Build history of the part. All positions in model axes, mm. Face numbers are marked on the shaded views. Give positions to 0.01 mm unless a question says otherwise; leave off trailing zeros. Order: outer loops, then holes, each group sorted by start corner. A loop starts at its lowest first (then second) coordinate and runs counter-clockwise, first axis right, second up. Notation, with made-up numbers: (5, 58.5) -> (51, 58.5) arc R23 cw to (51, 97.5) -> close; hole circle Ø7 at (81, 52). An arc over 180 degrees is marked (long way). One line per question, with ' | ' between items. Start each with the question number.
(1) Pull direction Z, two halves, no side cores. Call the marked faces 1 and 2: +Z half, -Z half, draft (parallel to the pull), parting line (faces both ways), or undercut.
(2) Cut at A-A (y = 8.5). Give the cut face in (x, z), then the cut area to 3 significant figures.
(3) Cut at C-C (y = 17). Give the cut face in (x, z).
(4) Cut at D-D (z = -20). Give the cut face in (x, y), then the cut area to 3 significant figures.
(5) Drill centre lines: L1, parallel to X at y = 6.5, z = -35.5; L2, parallel to Z at x = -18, y = 4; L3, parallel to X at y = 18.5, z = -81. Where is each one in solid material? Low to high. Write a range as from..to.
(6) Cut at B-B (x = -71). Give the cut face in (y, z).
(7) Pin check, flat tips, straight feed: pin 1 Ø3 at (x, y) = (-17.5, 5.5) entering from +Z; pin 2 Ø10 at (y, z) = (22, -104) entering from +X; pin 3 Ø1.9 at (x, z) = (-84, -85) entering from +Y. Stop position of each tip, or through.
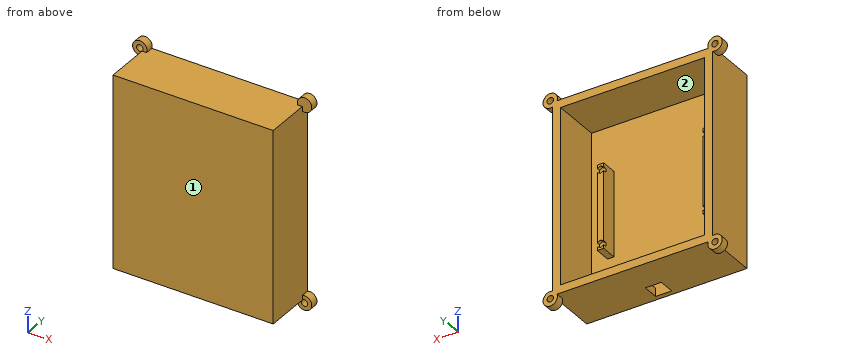
Autodesk Inventor part; units mm, degrees
ref_plane "YZ Plane" through (0, 0, 0) normal (1, 0, 0) x (0, 1, 0)
ref_plane "XZ Plane" through (0, 0, 0) normal (0, 1, 0) x (-1, 0, 0)
ref_plane "XY Plane" through (0, 0, 0) normal (0, 0, 1) x (1, 0, 0)
sketch "Sketch2" plane through (0, 0, 0) normal (0, 1, 0) x (-1, 0, 0)
  line L0 (0, 0) -> (100, 0)
  line L1 (100, 0) -> (100, -120)
  line L2 (100, -120) -> (0, -120)
  line L3 (0, -120) -> (0, 0)
  dimension "d0" = 100
  dimension "d1" = 120
extrude "Extrusion1" add sketch "Sketch2" along normal blind 3
sketch "Sketch3" plane through (0, 3, 0) normal (0, 1, 0) x (1, 0, 0)
  line L0 (0, 120) -> (-100, 120)
  line L1 (-100, 120) -> (-100, 0)
  line L2 (-95, 115) -> (-5, 115)
  line L3 (-5, 115) -> (-5, 5)
  line L4 (-5, 5) -> (-95, 5)
  line L5 (-95, 5) -> (-95, 115)
  line L6 (-100, 120) -> (0, 120)
  line L7 (0, 120) -> (0, 0)
  line L8 (0, 0) -> (-100, 0)
  line L9 (-100, 0) -> (-100, 120)
  dimension "d6" = 90
  dimension "d7" = 110
extrude "Extrusion2" add sketch "Sketch3" along normal blind 30
sketch "Sketch4" plane through (0, 3, 0) normal (0, 1, 0) x (1, 0, 0)
  line L0 (-95, 115) -> (-95, 5)
  line L1 (-95, 115) -> (-95, 85)
  line L2 (-85, 85) -> (-15, 85)
  line L3 (-15, 85) -> (-15, 35)
  line L4 (-15, 35) -> (-85, 35)
  line L5 (-85, 35) -> (-85, 85)
  line L6 (-85, 85) -> (-81, 85)
  line L7 (-81, 85) -> (-81, 35)
  line L8 (-81, 35) -> (-85, 35)
  line L9 (-85, 35) -> (-85, 85)
  line L10 (-15, 85) -> (-19, 85)
  line L11 (-19, 85) -> (-19, 35)
  line L12 (-19, 35) -> (-15, 35)
  line L13 (-15, 35) -> (-15, 85)
  line L14 (-85, 85) -> (-81, 85)
  line L15 (-81, 85) -> (-81, 81)
  line L16 (-81, 81) -> (-85, 81)
  line L17 (-85, 81) -> (-85, 85)
  line L18 (-85, 35) -> (-81, 35)
  line L19 (-81, 35) -> (-81, 39)
  line L20 (-81, 39) -> (-85, 39)
  line L21 (-85, 39) -> (-85, 35)
  line L22 (-19, 35) -> (-15, 35)
  line L23 (-15, 35) -> (-15, 39)
  line L24 (-15, 39) -> (-19, 39)
  line L25 (-19, 39) -> (-19, 35)
  line L26 (-19, 85) -> (-15, 85)
  line L27 (-15, 85) -> (-15, 81)
  line L28 (-15, 81) -> (-19, 81)
  line L29 (-19, 81) -> (-19, 85)
  circle A0 centre (-83, 83) radius 1
  circle A1 centre (-83, 37) radius 1
  circle A2 centre (-17, 37) radius 1
  circle A3 centre (-17, 83) radius 1
  point P0 (0, 0)
  dimension "d12" = 70
  dimension "d13" = 50
  dimension "d14" = 4
  dimension "d15" = 4
  dimension "d16" = 4
  dimension "d17" = 4
  dimension "d18" = 2
  dimension "d19" = 2
  dimension "d20" = 2
sketch "Sketch5" plane through (0, 33, 0) normal (0, 1, 0) x (1, 0, 0)
  point P0 (0, 0)
sketch "Sketch6" plane through (0, 33, 0) normal (0, 1, 0) x (1, 0, 0)
  line L0 (-100, 0) -> (0, 0)
  line L1 (0, 0) -> (10, 0) construction
  circle A0 centre (1.4142, -1.4142) radius 2
  circle A1 centre (1.4142, -1.4142) radius 4.5
  circle A2 centre (1.4084, 121.4127) radius 2
  circle A3 centre (1.4084, 121.4127) radius 4.5
  circle A4 centre (-101.4585, 121.4298) radius 2
  circle A5 centre (-101.4585, 121.4298) radius 4.5
  circle A6 centre (-101.4195, -1.4184) radius 2
  circle A7 centre (-101.4195, -1.4184) radius 4.5
  dimension "d24" = 4
  dimension "d25" = 9
  dimension "d27" = 4
  dimension "d28" = 9
  dimension "d30" = 4
  dimension "d31" = 9
  dimension "d33" = 4
  dimension "d34" = 9
extrude "Extrusion3" add sketch "Sketch6" against normal blind 5
extrude "Extrusion4" add sketch "Sketch4" along normal blind 10 contours L16 L7 L20 L5 | L28 L3 L24 L11
sketch "Sketch7" plane through (0, 13, 0) normal (0, 1, 0) x (1, 0, 0)
  point P0 (0, 0)
sketch "Sketch10" plane through (0, 13, 0) normal (0, 1, 0) x (1, 0, 0)
  line L0 (-81, 81) -> (-85, 81)
  line L1 (-81, 39) -> (-81, 81)
  line L2 (-85, 81) -> (-81, 81)
  line L3 (-81, 81) -> (-81, 39)
  line L4 (-81, 39) -> (-85, 39)
  line L5 (-85, 39) -> (-85, 81)
  point P0 (0, 0)
sketch "Sketch11" plane through (0, 13, 0) normal (0, 1, 0) x (1, 0, 0)
  line L0 (-15, 81) -> (-19, 81)
  line L1 (-15, 39) -> (-15, 81)
  line L2 (-19, 81) -> (-15, 81)
  line L3 (-15, 81) -> (-15, 39)
  line L4 (-15, 39) -> (-19, 39)
  line L5 (-19, 39) -> (-19, 81)
  line L6 (-85, 81) -> (-81, 81)
  line L7 (-85, 81) -> (-81, 81)
  line L8 (-81, 81) -> (-81, 85)
  line L9 (-81, 85) -> (-85, 85)
  line L10 (-85, 85) -> (-85, 81)
  line L11 (-19, 39) -> (-19, 81)
  line L12 (-19, 81) -> (-15, 81)
  line L13 (-15, 81) -> (-15, 85)
  line L14 (-15, 85) -> (-19, 85)
  line L15 (-19, 85) -> (-19, 81)
  line L16 (-15, 39) -> (-19, 39)
  line L17 (-19, 39) -> (-15, 39)
  line L18 (-15, 39) -> (-15, 35)
  line L19 (-15, 35) -> (-19, 35)
  line L20 (-19, 35) -> (-19, 39)
  line L21 (-85, 39) -> (-81, 39)
  line L22 (-81, 39) -> (-81, 35)
  line L23 (-81, 35) -> (-85, 35)
  line L24 (-85, 35) -> (-85, 39)
  circle A0 centre (-83, 83) radius 1
  circle A1 centre (-17, 83) radius 1
  circle A2 centre (-17, 37) radius 1
  circle A3 centre (-83, 37) radius 1
  line L25 (-19, 84.1547) -> (-17, 85.3094)
  line L26 (-17, 85.3094) -> (-15, 84.1547)
  line L27 (-15, 84.1547) -> (-15, 81.8453)
  line L28 (-15, 81.8453) -> (-17, 80.6906)
  line L29 (-17, 80.6906) -> (-19, 81.8453)
  line L30 (-19, 81.8453) -> (-19, 84.1547)
  line L31 (-19, 38.1547) -> (-17, 39.3094)
  line L32 (-17, 39.3094) -> (-15, 38.1547)
  line L33 (-15, 38.1547) -> (-15, 35.8453)
  line L34 (-15, 35.8453) -> (-17, 34.6906)
  line L35 (-17, 34.6906) -> (-19, 35.8453)
  line L36 (-19, 35.8453) -> (-19, 38.1547)
  line L37 (-81, 35.8453) -> (-83, 34.6906)
  line L38 (-83, 34.6906) -> (-85, 35.8453)
  line L39 (-85, 35.8453) -> (-85, 38.1547)
  line L40 (-85, 38.1547) -> (-83, 39.3094)
  line L41 (-83, 39.3094) -> (-81, 38.1547)
  line L42 (-81, 38.1547) -> (-81, 35.8453)
  line L43 (-81, 81.8453) -> (-83, 80.6906)
  line L44 (-83, 80.6906) -> (-85, 81.8453)
  line L45 (-85, 81.8453) -> (-85, 84.1547)
  line L46 (-85, 84.1547) -> (-83, 85.3094)
  line L47 (-83, 85.3094) -> (-81, 84.1547)
  line L48 (-81, 84.1547) -> (-81, 81.8453)
  point P0 (0, 0)
  point P1 (-19, 83)
  point P2 (-19, 37)
  point P3 (-81, 37)
  point P4 (-81, 83)
  dimension "d75" = 4
  dimension "d76" = 4
  dimension "d77" = 2
  dimension "d78" = 2
  dimension "d79" = 2
sketch "Sketch17" plane through (0, 3, 0) normal (0, 1, 0) x (1, 0, 0)
  line L0 (-85, 85) -> (-15, 85)
  line L1 (-15, 85) -> (-15, 35)
  line L2 (-15, 35) -> (-85, 35)
  line L3 (-85, 35) -> (-85, 85)
  line L4 (-85, 85) -> (-81, 85)
  line L5 (-81, 85) -> (-81, 35)
  line L6 (-81, 35) -> (-85, 35)
  line L7 (-85, 35) -> (-85, 85)
  line L8 (-15, 85) -> (-19, 85)
  line L9 (-19, 85) -> (-19, 35)
  line L10 (-19, 35) -> (-15, 35)
  line L11 (-15, 35) -> (-15, 85)
  point P0 (0, 0)
  point P1 (-95, 115)
extrude "Extrusion7" add sketch "Sketch17" along normal blind 10 contours L0 L5 L2 L3 | L0 L1 L2 L9
sketch "Sketch18" plane through (0, 3, 0) normal (0, 1, 0) x (1, 0, 0)
  line L0 (-19, 35) -> (-19, 85)
  line L1 (-19, 35) -> (-15, 35)
  line L2 (-15, 35) -> (-15, 33.5)
  line L3 (-15, 33.5) -> (-19, 33.5)
  line L4 (-19, 33.5) -> (-19, 35)
  line L5 (-19, 85) -> (-15, 85)
  line L6 (-15, 85) -> (-15, 86.5)
  line L7 (-15, 86.5) -> (-19, 86.5)
  line L8 (-19, 86.5) -> (-19, 85)
  line L9 (-81, 85) -> (-85, 85)
  line L10 (-85, 85) -> (-81, 85)
  line L11 (-81, 85) -> (-81, 86.5)
  line L12 (-81, 86.5) -> (-85, 86.5)
  line L13 (-85, 86.5) -> (-85, 85)
  line L14 (-85, 35) -> (-81, 35)
  line L15 (-85, 35) -> (-81, 35)
  line L16 (-81, 35) -> (-81, 33.5)
  line L17 (-81, 33.5) -> (-85, 33.5)
  line L18 (-85, 33.5) -> (-85, 35)
  point P0 (0, 0)
  dimension "d80" = 4
  dimension "d81" = 1.5
  dimension "d82" = 1.5
extrude "Extrusion8" add sketch "Sketch18" along normal blind 10
extrude "Extrusion9" cut sketch "Sketch11" against normal blind 2 contours L28 L29 L0 | L0 L29 L15 L25 L14 L26 L13 L28 | L32 L18 L34 L19 L35 L20 L31 L4 | L4 L31 L32 | L14 L25 L26 | L34 L35 L19 | L44 L10 L46 L9 L47 L8 L43 L6 | L6 L43 L44 | L46 L47 L9 | L40 L41 L21 | L21 L41 L22 L37 L23 L38 L24 L40 | L23 L37 L38 | A0 | A1 | A2 | A3
sketch "Sketch19" plane through (0, 28, 0) normal (0, -1, 0) x (1, 0, 0)
  circle A0 centre (1.4142, 1.4142) radius 2
  circle A1 centre (1.4142, 1.4142) radius 2
  circle A2 centre (1.4142, 1.4142) radius 4.5
  circle A3 centre (-101.4195, 1.4184) radius 2
  circle A4 centre (-101.4195, 1.4184) radius 2
  circle A5 centre (-101.4195, 1.4184) radius 4.5
  circle A6 centre (-101.4585, -121.4298) radius 2
  circle A7 centre (-101.4585, -121.4298) radius 2
  circle A8 centre (-101.4585, -121.4298) radius 4.5
  circle A9 centre (1.4142, -121.4298) radius 2.0171
  arc A10 (-0.0073, -120) -> (0, -119.9927) centre (1.4084, -121.4127) ccw
  circle A11 centre (1.4084, -121.4127) radius 4.5
  point P0 (0, 0)
sketch "Sketch20" plane through (0, 0, -120) normal (0, 0, -1) x (-1, 0, 0)
  line L0 (100, 28) -> (100, 33)
  line L1 (0, 0) -> (100, 0)
  line L2 (100, 0) -> (100, 33)
  line L3 (100, 33) -> (0, 33)
  line L4 (0, 33) -> (0, 0)
  line L5 (95, 3) -> (5, 3)
  line L6 (50, 3) -> (55, 3)
  line L7 (55, 3) -> (55, 13)
  line L8 (55, 13) -> (50, 13)
  line L9 (50, 13) -> (45, 13)
  line L10 (45, 13) -> (45, 3)
  line L11 (45, 3) -> (50, 3)
  line L12 (55, 13) -> (45, 13)
  line L13 (45, 13) -> (45, 3)
  line L14 (45, 3) -> (55, 3)
  line L15 (55, 3) -> (55, 13)
extrude "Extrusion10" cut sketch "Sketch20" against normal blind 10 contours L5 L10 L9 L8 L7
properties part number "Spod"
Result set:
1) face 1: draft | face 2: undercut
2) outline: (-100, -120) -> (-55, -120) -> (-55, -115) -> (-95, -115) -> (-95, -5) -> (-5, -5) -> (-5, -115) -> (-45, -115) -> (-45, -120) -> (0, -120) -> (0, 0) -> (-100, 0) -> close; (-85, -86.5) -> (-81, -86.5) -> (-81, -33.5) -> (-85, -33.5) -> close; (-19, -86.5) -> (-15, -86.5) -> (-15, -33.5) -> (-19, -33.5) -> close | area: 2,470 mm2
3) outline: (-100, -120) -> (0, -120) -> (0, 0) -> (-100, 0) -> close; hole (-95, -115) -> (-5, -115) -> (-5, -5) -> (-95, -5) -> close
4) outline: (-100, 0) -> (0, 0) -> (0, 33) -> (-5, 33) -> (-5, 3) -> (-95, 3) -> (-95, 33) -> (-100, 33) -> close | area: 600 mm2
5) L1: x = -100..-95, -85..-81, -19..-15, -5..0 | L2: z = -120..-115, -86.5..-33.5, -5..0 | L3: x = -100..-95, -5..0
6) outline: (0, -120) -> (33, -120) -> (33, -115) -> (3, -115) -> (3, -5) -> (33, -5) -> (33, 0) -> (0, 0) -> close
7) pin 1: stops at z = 0 | pin 2: stops at x = 0 | pin 3: stops at y = 13
